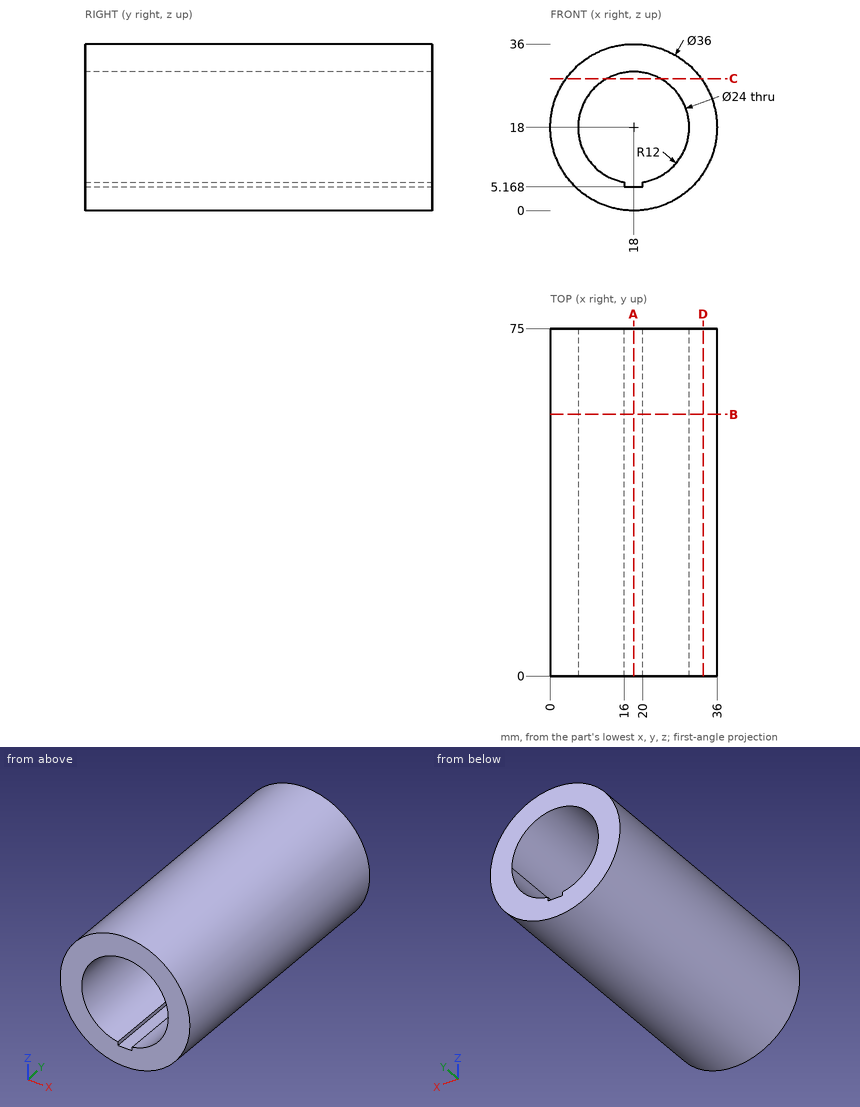
Job drawing, mm, ordinate dimensions from the low corner. One solid piece. Give positions to 0.01 mm unless a question says otherwise; leave off trailing zeros. Loops run counter-clockwise (first coordinate to the right, second up) from the corner with the lowest first, then second, coordinate; pieces in that order, holes last.
Item 1: Slice it at B-B, the plane y = 56.5. List the corners of the cut face in (x, z), and give its area (3 significant figures).
Answers follow:
outline: circle Ø36 at (18, 18); hole (16, 5.17) - (20, 5.17) - (20, 6.17) arc R12 ccw (long way) to (16, 6.17) - close
area: 562 mm2
Item 2: Flat gauge pins, fed straight in: pin 1 (2 mm diameter, centred on x = 7, y = 38.5, fed in from -Z); pin 2 (0.5 mm diameter, centred on y = 28.5, z = 6, fed in from +X); pin 3 (4 mm diameter, centred on x = 12.5, y = 64.5, fed in from -Z); pin 4 (3 mm diameter, centred on x = 26, z = 24, fed in from -Y). Where does each tip first touch, or does it go through?
Answers follow:
pin 1: stops at z = 3.03
pin 2: stops at x = 31.64
pin 3: stops at z = 0.34
pin 4: passes through
Item 3: Drill centre lines: line 1 (X direction, y = 34, z = 18); line 2 (Z direction, x = 18.5, y = 41.5); line 3 (X direction, y = 70, z = 22.5). Where is each one in solid material? Low to high.
Answers follow:
line 1: x = 0 to 6, 30 to 36
line 2: z = 0.01 to 5.17, 29.99 to 35.99
line 3: x = 0.57 to 6.88, 29.12 to 35.43
Item 4: Slice it at C-C, the plane z = 28.5. List the corners of the cut face in (x, y).
Answers follow:
outline: (3.38, 0) - (12.19, 0) - (12.19, 75) - (3.38, 75) - close; (23.81, 0) - (32.62, 0) - (32.62, 75) - (23.81, 75) - close
Item 5: Slice it at A-A, the plane x = 18. List the corners of the cut face in (y, z).
Answers follow:
outline: (0, 0) - (75, 0) - (75, 5.17) - (0, 5.17) - close; (0, 30) - (75, 30) - (75, 36) - (0, 36) - close
Item 6: Slice it at D-D, the plane x = 33. List the corners of the cut face in (y, z), and give its area (3 significant figures).
Answers follow:
outline: (0, 8.05) - (75, 8.05) - (75, 27.95) - (0, 27.95) - close
area: 1,490 mm2
